```python
from build123d import *

# Parameters (mm, degrees)
F0_W     = 101.6
F0_H     = 101.6
F1_DEPTH = 25.4
F2_SIZE  = 25.4
F3_T     = -2.54


with BuildPart() as f1:
    # F0 (on Front) → F1 (new body, symmetric)
    with BuildSketch(Plane.XZ):
        Rectangle(F0_W, F0_H)
    extrude(amount=F1_DEPTH, both=True)

    # F2
    f2_edges = [f1.edges().sort_by_distance(p)[0] for p in [
        (-50.8, 0, 50.8),
        (50.8, 0, 50.8),
        (-50.8, 0, -50.8),
        (50.8, 0, -50.8),
    ]]
    chamfer(f2_edges, length=F2_SIZE)

    # F3
    f3_openings = [f1.faces().sort_by_distance(p)[0] for p in [
        (0, -25.4, 0),
    ]]
    offset(amount=F3_T, openings=f3_openings)


solid = f1.part
```
For this review, take the finished solid that the model builds, in its own axes (mm). A direction names the side the tool comes from. Coordinates: 2 decimals unless noted, no trailing zeros. Write each loop counter-clockwise with the first axis right and the second up, starting at its lowest first coordinate (ties: lowest second). Pieces come first, ordered by that corner, then holes. Notation, with made-up numbers: (1.25, 7) - (47.25, 7) arc R28 cw to (47.25, 40) - close; hole circle Ø6 at (-15, 75.5). An arc over 180 degrees is marked (long way). Answer in a Markdown table with one row per item. Add a question column.
Q1. We need section C-C, the plane x = 10.5. State the section outline as (y, z) points.
Q2. We need section B-B, the plane z = -17. State the section outline as (x, y) points, and give its area (3 significant figures).
Q3. For P1, Ø1, axis at x = 29, y = -19, coming from the +Z side; P2, Ø8, axis at x = 18.5, z = -37.5, coming from the -Y side; P3, Ø4, axis at x = -33, y = 4, coming from the -Z side, all flat-tipped, find the tip position at first contact; note any pin that passes through.
Q4. For probe 1 along Z at (x, y) = (-9, 6); probe 2 along Y at (x, z) = (-35, -33.5), list the stretches that pass through material, from the lowest coordinate up.
Q5. We need section A-A, the plane y = -1. State the section outline as (x, z) points.
Q6. Draft analysis for pull direction X (two halves, no side actions). For faces 1 (the flat face through (-48.26, -2, 0)), 2 (the flat face through (0, 0, -50.8)), 3 (the flat face through (37.9, -0.4, 38.3)), state which applies: +X half, -X half, draft (parallel to the pull), parting line (faces both ways), or undercut.
Q7. Tool access review of faces 4 (the flat face through (-36.14, -1.61, 36.47)), 5 (the flat face through (-49, -25.4, 0)): name each direction out of +Z, -Z, +X, -X, +Y, -Y from which nothing blocks a thin tool from reaching the whole face with its end or side.
Answer list:
| question | item | result |
|---|---|---|
| 1 | outline | (-25.4, -50.8) - (25.4, -50.8) - (25.4, 50.8) - (-25.4, 50.8) - (-25.4, 48.26) - (22.86, 48.26) - (22.86, -48.26) - (-25.4, -48.26) - close |
| 2 | outline | (-50.8, -25.4) - (-48.26, -25.4) - (-48.26, 22.86) - (48.26, 22.86) - (48.26, -25.4) - (50.8, -25.4) - (50.8, 25.4) - (-50.8, 25.4) - close |
| 2 | area | 503 mm2 |
| 3 | P1 | stops at z = 47.7 |
| 3 | P2 | stops at y = 22.86 |
| 3 | P3 | stops at z = -45.2 |
| 4 | probe 1 | z = -50.8 to -48.26, 48.26 to 50.8 |
| 4 | probe 2 | y = 22.86 to 25.4 |
| 5 | outline | (-50.8, -25.4) - (-25.4, -50.8) - (25.4, -50.8) - (50.8, -25.4) - (50.8, 25.4) - (25.4, 50.8) - (-25.4, 50.8) - (-50.8, 25.4) - close; hole (-48.26, -24.35) - (-24.35, -48.26) - (24.35, -48.26) - (48.26, -24.35) - (48.26, 24.35) - (24.35, 48.26) - (-24.35, 48.26) - (-48.26, 24.35) - close |
| 6 | face 1 | undercut |
| 6 | face 2 | draft |
| 6 | face 3 | +X half |
| 7 | face 4 | -Y |
| 7 | face 5 | +Z, -Z, +X, -X, -Y |
